from build123d import *

# Parameters (mm, degrees)
SKETCH002_W                  = 85.5
SKETCH002_H                  = 67.5
PAD_DEPTH                    = 7.5
POCKET_DEPTH                 = 18
POCKET_LINEARPATTERN_2_DEPTH = 18
LINEARPATTERN001_COUNT       = 2
LINEARPATTERN001_PITCH       = 44
SKETCH003_W                  = 21
SKETCH003_H                  = 26
POCKET001_DEPTH              = 20
LINEARPATTERN002_COUNT       = 3
LINEARPATTERN002_PITCH       = 31
SKETCH004_W                  = 6.5
SKETCH004_H                  = 26
POCKET002_DEPTH              = 6
LINEARPATTERN003_COUNT       = 2
LINEARPATTERN003_PITCH       = 31
PAD001_DEPTH                 = 1
FILLET_R                     = 2


with BuildPart() as part:
    # Sketch002 → Pad (new body, symmetric)
    with BuildSketch(Plane.XZ):
        Rectangle(SKETCH002_W, SKETCH002_H)
    extrude(amount=PAD_DEPTH, both=True)

    # Sketch → Pocket (cut, symmetric)
    with BuildSketch(Plane(origin=(-22, 6, 24), x_dir=(0, 0, 1), z_dir=(1, 0, 0))):
        with BuildLine():
            ThreePointArc((-7.314507, 4.802134), (0, -8.75), (7.314507, 4.802134))
            ThreePointArc((7.314507, 4.802134), (4.058795, 8.698798), (0, 11.75))
            ThreePointArc((0, 11.75), (-4.058795, 8.698798), (-7.314507, 4.802134))
        make_face()
    pocket = extrude(amount=POCKET_DEPTH, both=True, mode=Mode.SUBTRACT)

    # Sketch LinearPattern 2 → Pocket LinearPattern 2 (cut, symmetric)
    with BuildSketch(Plane(origin=(-22, 6, 5), x_dir=(0, 0, 1), z_dir=(1, 0, 0))):
        with BuildLine():
            ThreePointArc((-7.314507, 4.802134), (0, -8.75), (7.314507, 4.802134))
            ThreePointArc((7.314507, 4.802134), (4.058795, 8.698798), (0, 11.75))
            ThreePointArc((0, 11.75), (-4.058795, 8.698798), (-7.314507, 4.802134))
        make_face()
    pocket_linearpattern_2 = extrude(amount=POCKET_LINEARPATTERN_2_DEPTH, both=True, mode=Mode.SUBTRACT)

    # LinearPattern001: Pocket, Pocket LinearPattern 2 ×2
    with Locations(*[(i * LINEARPATTERN001_PITCH, 0, 0) for i in range(1, LINEARPATTERN001_COUNT)]):
        add(pocket, mode=Mode.SUBTRACT)
        add(pocket_linearpattern_2, mode=Mode.SUBTRACT)

    # Sketch003 → Pocket001 (cut)
    with BuildSketch(Plane(origin=(-31, -7, -19), x_dir=(1, 0, 0), z_dir=(0, -1, 0))):
        Rectangle(SKETCH003_W, SKETCH003_H)
    pocket001 = extrude(amount=-POCKET001_DEPTH, mode=Mode.SUBTRACT)

    # LinearPattern002: Pocket001 ×3
    with Locations(*[(i * LINEARPATTERN002_PITCH, 0, 0) for i in range(1, LINEARPATTERN002_COUNT)]):
        add(pocket001, mode=Mode.SUBTRACT)

    # Sketch004 → Pocket002 (cut)
    with BuildSketch(Plane(origin=(15.5, 2, -19), x_dir=(1, 0, 0), z_dir=(0, -1, 0))):
        Rectangle(SKETCH004_W, SKETCH004_H)
    pocket002 = extrude(amount=-POCKET002_DEPTH, mode=Mode.SUBTRACT)

    # LinearPattern003: Pocket002 ×2
    with Locations(*[(-i * LINEARPATTERN003_PITCH, 0, 0) for i in range(1, LINEARPATTERN003_COUNT)]):
        add(pocket002, mode=Mode.SUBTRACT)

    # Sketch005 → Pad001 (join, symmetric)
    with BuildSketch(Plane.YZ):
        with BuildLine():
            ThreePointArc((19, 23), (9, 33), (-1, 23))
            Line((-1, 23), (-1, 5))
            ThreePointArc((-1, 5), (9, -5), (19, 5))
            Line((19, 23), (19, 5))
        make_face()
    extrude(amount=PAD001_DEPTH, both=True)

    # Fillet
    fillet_edges = [part.edges().sort_by_distance(p)[0] for p in [
        (0, -7.5, 33.75),
        (42.75, -7.5, 0),
        (0, -7.5, -33.75),
        (-42.75, -7.5, 0),
    ]]
    fillet(fillet_edges, radius=FILLET_R)


solid = part.part
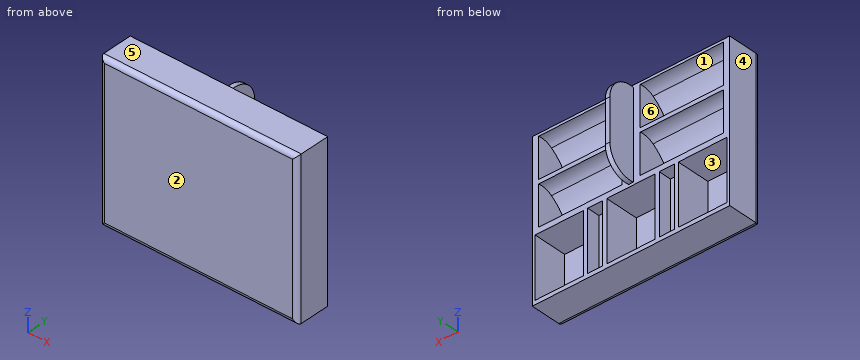
The model under review builds one solid part; all positions refer to its coordinate system, in mm. Face numbers are marked on the shaded views. A direction names the side the tool comes from. Give positions to 0.01 mm unless a question says otherwise; leave off trailing zeros. Loops run counter-clockwise (first coordinate to the right, second up) from the corner with the lowest first, then second, coordinate; pieces in that order, holes last. Notation, with made-up numbers: (-33, 51.5) -> (-11, 51.5) arc R24 ccw to (-11, 89.5) -> close; hole circle Ø6 at (77.5, 38.5). An arc over 180 degrees is marked (long way). Put each result on its own line as item: value. Start each with the question number.
1. We need section D-D on y = 9. State the section outline as (x, z) points.
2. We need section A-A on y = -3. State how many separate pieces and enclosed holes the cut face has, then the cut area to 3 significant figures.
3. For the marked faces 1, 2 and 3, list the 3-axis set-ups (+Z, -Z, +X, -X, +Y, -Y) from which the entire face can be reached by the end or side of a thin tool; tool diameter is ignored.
4. Clearance check with flat-ended pins moving along their axes: P1, Ø3.5, axis at y = 13.5, z = 11, coming from the -X side; P2, Ø6, axis at x = 7.5, z = 26.5, coming from the +Y side; P3, Ø17, axis at x = 33.5, z = -18, coming from the +Y side. State where each tip first meets the part, or that it passes through.
5. Mouldability with a two-part tool opening along X and no side actions: class the marked faces 4, 5 and 6 as released by +X, released by -X, zero draft, split by the parting line, or undercut.
6. We need section B-B on x = -2.5. State the section outline as (y, z) points.
7. Wall thickness on probe 1 along Z at (x, y) = (-9, 6.25); probe 2 along X at (y, z) = (2.5, -12.5); probe 3 along X at (y, z) = (3.25, 13): over which ranges is each line inside the solid? List them lowest first.
8. We need section C-C on z = -20. State the section outline as (x, y) points.
Determined:
1. outline: (-1, -5) -> (1, -5) -> (1, 33) -> (-1, 33) -> close
2. separate pieces: 1
2. enclosed holes: 7
2. area: 3,060 mm^2
3. face 1: none
3. face 2: +Z, -Z, +X, -X, -Y
3. face 3: +Y
4. P1: x = -1
4. P2: y = -1.19
4. P3: y = 7.5
5. face 4: released by -X
5. face 5: zero draft
5. face 6: undercut
6. outline: (-7.5, -31.75) arc R2 ccw to (-5.5, -33.75) -> (7.5, -33.75) -> (7.5, -32) -> (-7, -32) -> (-7, -6) -> (7.5, -6) -> (7.5, 33.75) -> (-5.5, 33.75) arc R2 ccw to (-7.5, 31.75) -> close
7. probe 1: -33.75 to -32, -6 to -3.75, 13.75 to 15.25, 32.75 to 33.75
7. probe 2: -42.75 to -41.5, -20.5 to -18.75, -12.25 to -10.5, 10.5 to 12.25, 18.75 to 20.5, 41.5 to 42.75
7. probe 3: -42.75 to -40, -4 to 4, 40 to 42.75
8. outline: (-42.75, -5.5) arc R2 ccw to (-40.75, -7.5) -> (40.75, -7.5) arc R2 ccw to (42.75, -5.5) -> (42.75, 7.5) -> (41.5, 7.5) -> (41.5, -7) -> (20.5, -7) -> (20.5, 7.5) -> (18.75, 7.5) -> (18.75, 2) -> (12.25, 2) -> (12.25, 7.5) -> (10.5, 7.5) -> (10.5, -7) -> (-10.5, -7) -> (-10.5, 7.5) -> (-12.25, 7.5) -> (-12.25, 2) -> (-18.75, 2) -> (-18.75, 7.5) -> (-20.5, 7.5) -> (-20.5, -7) -> (-41.5, -7) -> (-41.5, 7.5) -> (-42.75, 7.5) -> close
